from build123d import *

# Parameters (mm, degrees)
SKETCH1_W           = 20
SKETCH1_H           = 10
BOSS_EXTRUDE1_DEPTH = 1.5
SKETCH3_W           = 5
SKETCH3_H           = 1.5
CUT_EXTRUDE1_DEPTH  = 2
SKETCH2_R           = 1
CUT_EXTRUDE2_DEPTH  = 2


with BuildPart() as part:
    # Sketch1 → Boss-Extrude1 (new body)
    with BuildSketch(Plane(origin=(0, 0, 0), x_dir=(1, 0, 0), z_dir=(0, 1, 0))):
        with Locations((2.275132275, -0.37037037)):
            Rectangle(SKETCH1_W, SKETCH1_H)
    extrude(amount=BOSS_EXTRUDE1_DEPTH)

    # Sketch3 → Cut-Extrude1 (cut)
    with BuildSketch(Plane(origin=(0, 1.5, 0), x_dir=(1, 0, 0), z_dir=(0, 1, 0))):
        with Locations((-2.724867725, 1.37962963)):
            Rectangle(SKETCH3_W, SKETCH3_H)
        with Locations((7.275132275, 1.37962963)):
            Rectangle(SKETCH3_W, SKETCH3_H)
        with Locations((7.275132275, -2.12037037)):
            Rectangle(SKETCH3_W, SKETCH3_H)
        with Locations((-2.724867725, -2.12037037)):
            Rectangle(SKETCH3_W, SKETCH3_H)
    extrude(amount=-CUT_EXTRUDE1_DEPTH, mode=Mode.SUBTRACT)

    # Sketch2 → Cut-Extrude2 (cut)
    with BuildSketch(Plane(origin=(0, 1.5, 0), x_dir=(1, 0, 0), z_dir=(0, 1, 0))):
        with Locations((2.275132275, -0.37037037)):
            Circle(SKETCH2_R)
    extrude(amount=-CUT_EXTRUDE2_DEPTH, mode=Mode.SUBTRACT)


solid = part.part
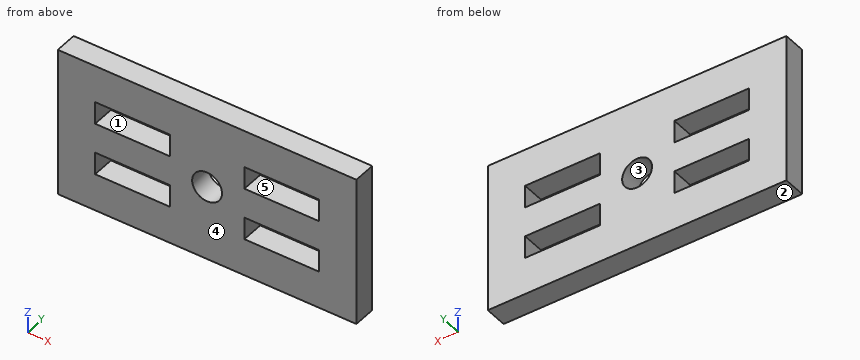
Here's how the part is built. I have some questions about the finished solid (model axes, mm). Face numbers are marked on the shaded views. A direction names the side the tool comes from. Round coordinates to 2 decimals unless told otherwise and drop trailing zeros. Loops run counter-clockwise (first coordinate to the right, second up) from the corner with the lowest first, then second, coordinate; pieces in that order, holes last. Notation, with made-up numbers: (78.25, 72.25) - (123.25, 72.25) arc R29 cw to (123.25, 92.25) - close; hole circle Ø7 at (-17, 17.5). An arc over 180 degrees is marked (long way). One line per question, with ' | ' between items. Start each with the question number.
Q1. I want a section at C-C (x = 2). Write out the boundary of the cut face in (y, z), then the cut area to 3 significant figures.
Q2. For the marked faces 1 and 2, which set-ups out of +Z, -Z, +X, -X, +Y, -Y let a thin tool reach every point of the face, with its end or its side?
Q3. I want a section at B-B (z = 0.75). Write out the boundary of the cut face in (x, y), then the cut area to 3 significant figures.
Q4. I want a section at D-D (y = 1.15). Write out the boundary of the cut face in (x, z), then the cut area to 3 significant figures.
Q5. Please list where these lines run through material, in increasing order: line 1 (X direction, y = 0.55, z = -1.75); line 2 (Z direction, x = -0.75, y = 0.3); line 3 (X direction, y = 0.8, z = -0.5). Write a range as [from, to].
Q6. We'd pull the mould along X, two halves only. Please class the marked faces 3, 4 and 5: +X half, -X half, draft (parallel to the pull), parting line (faces both ways), or undercut.
Q7. I want a section at A-A (x = -1). Write out the boundary of the cut face in (y, z), then the cut area to 3 significant figures.
Response values:
1) outline: (0, -4.63) - (1.5, -4.63) - (1.5, -0.59) - (0, -0.59) - close; (0, 1.33) - (1.5, 1.33) - (1.5, 5.37) - (0, 5.37) - close | area: 12.1 mm²
2) face 1: +Y, -Y | face 2: -Z, +X, -X, +Y, -Y
3) outline: (-7.72, 0) - (1.35, 0) - (1.35, 1.5) - (-7.72, 1.5) - close; (3.2, 0) - (12.28, 0) - (12.28, 1.5) - (3.2, 1.5) - close | area: 27.2 mm²
4) outline: (-7.72, -4.63) - (12.28, -4.63) - (12.28, 5.37) - (-7.72, 5.37) - close; hole (-5.22, -2.13) - (-0.22, -2.13) - (-0.22, -0.63) - (-5.22, -0.63) - close; hole (-5.22, 1.37) - (-0.22, 1.37) - (-0.22, 2.87) - (-5.22, 2.87) - close; hole circle Ø2 at (2.28, 0.37); hole (4.78, -2.13) - (9.78, -2.13) - (9.78, -0.63) - (4.78, -0.63) - close; hole (4.78, 1.37) - (9.78, 1.37) - (9.78, 2.87) - (4.78, 2.87) - close | area: 167 mm²
5) line 1: x = [-7.72, -5.22], [-0.22, 4.78], [9.78, 12.28] | line 2: z = [-4.63, -2.13], [-0.63, 1.37], [2.87, 5.37] | line 3: x = [-7.72, 1.78], [2.77, 12.28]
6) face 3: undercut | face 4: draft | face 5: undercut
7) outline: (0, -4.63) - (1.5, -4.63) - (1.5, -2.13) - (0, -2.13) - close; (0, -0.63) - (1.5, -0.63) - (1.5, 1.37) - (0, 1.37) - close; (0, 2.87) - (1.5, 2.87) - (1.5, 5.37) - (0, 5.37) - close | area: 10.5 mm²
